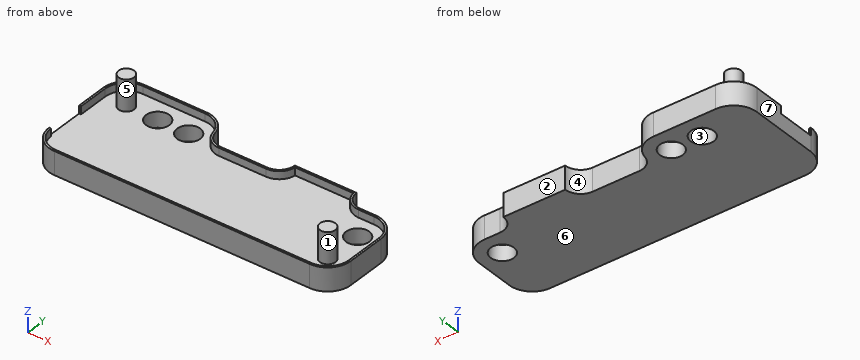
from build123d import *

# Parameters (mm, degrees)
SKETCH1_R           = 1
SKETCH1_R_2         = 1.5
BOSS_EXTRUDE1_DEPTH = 2
BOSS_EXTRUDE2_DEPTH = 3
SKETCH1_4_R         = 1
BOSS_EXTRUDE3_DEPTH = 6
SKETCH2_W           = 4
SKETCH2_H           = 5
CUT_EXTRUDE1_DEPTH  = 3


with BuildPart() as part:
    # Sketch1 → Boss-Extrude1 (new body)
    with BuildSketch(Plane.XY):
        with BuildLine():
            ThreePointArc((3, 0.25), (1.055456352, 1.055456352), (0.25, 3))
            Line((0.25, 3), (0.25, 12))
            ThreePointArc((0.25, 12), (1.055456352, 13.944543648), (3, 14.75))
            Line((3, 14.75), (11.060612309, 14.75))
            ThreePointArc((11.060612309, 14.75), (12.799865022, 14.13014084), (13.755051026, 12.55))
            ThreePointArc((13.755051026, 12.55), (14.536566847, 11.257157494), (15.959591794, 10.75))
            Line((15.959591794, 10.75), (22, 10.75))
            ThreePointArc((22, 10.75), (23.5, 11.322949017), (24.236067977, 12.75))
            Line((24.236067977, 12.75), (31.763932023, 12.75))
            ThreePointArc((31.763932023, 12.75), (32.5, 11.322949017), (34, 10.75))
            Line((34, 10.75), (36, 10.75))
            ThreePointArc((36, 10.75), (37.944543648, 9.944543648), (38.75, 8))
            Line((38.75, 8), (38.75, 3))
            ThreePointArc((38.75, 3), (37.944543648, 1.055456352), (36, 0.25))
            Line((36, 0.25), (3, 0.25))
        make_face()
        with Locations((36, 3)):
            Circle(SKETCH1_R, mode=Mode.SUBTRACT)
        with Locations((36, 8)):
            Circle(SKETCH1_R_2, mode=Mode.SUBTRACT)
        with Locations((3, 12)):
            Circle(SKETCH1_R, mode=Mode.SUBTRACT)
        with Locations((7.060612309, 12)):
            Circle(SKETCH1_R_2, mode=Mode.SUBTRACT)
        with Locations((11.060612309, 12)):
            Circle(SKETCH1_R_2, mode=Mode.SUBTRACT)
    extrude(amount=BOSS_EXTRUDE1_DEPTH)

    # Sketch1_3 → Boss-Extrude2 (add)
    with BuildSketch(Plane.XY):
        with BuildLine():
            Line((3, 0), (36, 0))
            ThreePointArc((36, 0), (38.121320344, 0.878679656), (39, 3))
            Line((39, 3), (39, 8))
            ThreePointArc((39, 8), (38.121320344, 10.121320344), (36, 11))
            Line((36, 11), (34, 11))
            ThreePointArc((34, 11), (32.585786438, 11.585786438), (32, 13))
            Line((32, 13), (24, 13))
            ThreePointArc((24, 13), (23.414213562, 11.585786438), (22, 11))
            Line((22, 11), (15.959591794, 11))
            ThreePointArc((15.959591794, 11), (14.69468073, 11.450806662), (14, 12.6))
            ThreePointArc((14, 12.6), (12.957978905, 14.323790008), (11.060612309, 15))
            Line((11.060612309, 15), (3, 15))
            ThreePointArc((3, 15), (0.878679656, 14.121320344), (0, 12))
            Line((0, 12), (0, 3))
            ThreePointArc((0, 3), (0.878679656, 0.878679656), (3, 0))
        make_face()
        with BuildLine():
            Line((3, 0.25), (36, 0.25))
            ThreePointArc((36, 0.25), (37.944543648, 1.055456352), (38.75, 3))
            Line((38.75, 3), (38.75, 8))
            ThreePointArc((38.75, 8), (37.944543648, 9.944543648), (36, 10.75))
            Line((36, 10.75), (34, 10.75))
            ThreePointArc((34, 10.75), (32.5, 11.322949017), (31.763932023, 12.75))
            Line((31.763932023, 12.75), (24.236067977, 12.75))
            ThreePointArc((24.236067977, 12.75), (23.5, 11.322949017), (22, 10.75))
            Line((22, 10.75), (15.959591794, 10.75))
            ThreePointArc((15.959591794, 10.75), (14.536566847, 11.257157494), (13.755051026, 12.55))
            ThreePointArc((13.755051026, 12.55), (12.799865022, 14.13014084), (11.060612309, 14.75))
            Line((11.060612309, 14.75), (3, 14.75))
            ThreePointArc((3, 14.75), (1.055456352, 13.944543648), (0.25, 12))
            Line((0.25, 12), (0.25, 3))
            ThreePointArc((0.25, 3), (1.055456352, 1.055456352), (3, 0.25))
        make_face(mode=Mode.SUBTRACT)
    extrude(amount=BOSS_EXTRUDE2_DEPTH)

    # Sketch1_4 → Boss-Extrude3 (add)
    with BuildSketch(Plane.XY):
        with Locations((3, 12)):
            Circle(SKETCH1_4_R)
        with Locations((36, 3)):
            Circle(SKETCH1_4_R)
    extrude(amount=BOSS_EXTRUDE3_DEPTH)

    # Sketch2 → Cut-Extrude1 (cut, symmetric)
    with BuildSketch(Plane.ZY):
        with Locations((4, 5.5)):
            Rectangle(SKETCH2_W, SKETCH2_H)
    extrude(amount=CUT_EXTRUDE1_DEPTH, both=True, mode=Mode.SUBTRACT)


solid = part.part
Input: part model. Units: mm. Frame: model coordinates. Face numbers are marked on the shaded views. A direction names the side the tool comes from. Round coordinates to 2 decimals unless told otherwise and drop trailing zeros. Order: outer loops, then holes, each group sorted by start corner. A loop starts at its lowest first (then second) coordinate and runs counter-clockwise, first axis right, second up.
1. Material intervals for line 1 (Y direction, x = 36, z = 2.5); line 2 (Y direction, x = 2.5, z = 2.5); line 3 (Y direction, x = 34.5, z = 2.45), sorted ascending.
The answers:
line 1: y = 0 to 0.25, 2 to 4, 10.75 to 11
line 2: y = 0.04 to 0.3, 11.13 to 12.87, 14.7 to 14.96
line 3: y = 0 to 0.25, 10.75 to 11
2. Mould query, pull axis X, two halves, no side actions, for the marked faces 5, 6 and 7. Classes: released by +X, released by -X, zero draft, split by the parting line, or undercut.
The answers:
face 5: undercut
face 6: zero draft
face 7: released by -X
3. Cut plane A-A, the plane z = 1.25. Output: boundary loops of the cut face in (x, y).
The answers:
outline: (0, 3) arc R3 ccw to (3, 0) - (36, 0) arc R3 ccw to (39, 3) - (39, 8) arc R3 ccw to (36, 11) - (34, 11) arc R2 cw to (32, 13) - (24, 13) arc R2 cw to (22, 11) - (15.96, 11) arc R2 cw to (14, 12.6) arc R3 ccw to (11.06, 15) - (3, 15) arc R3 ccw to (0, 12) - close; hole circle Ø3 at (7.06, 12); hole circle Ø3 at (11.06, 12); hole circle Ø3 at (36, 8)
4. Cut plane B-B, the plane x = 26.5. Output: boundary loops of the cut face in (y, z).
The answers:
outline: (0, 0) - (13, 0) - (13, 3) - (12.75, 3) - (12.75, 2) - (0.25, 2) - (0.25, 3) - (0, 3) - close
5. Pin query (flat end, axial travel): P1, Ø0.9, axis at x = 18.5, z = 2, coming from the +Y side; P2, Ø4, axis at x = 11.06, y = 12, coming from the +Z side; P3, Ø1, axis at x = 21.5, z = 5, coming from the -Y side; P4, Ø7.5, axis at x = 12, y = 9, coming from the +Z side. Return the tip coordinate at first contact, or that it passes through.
The answers:
P1: stops at y = 11
P2: stops at z = 2
P3: passes through
P4: stops at z = 3
6. Cut plane D-D, the plane z = 3.4. Output: boundary loops of the cut face in (x, y).
The answers:
outline: circle Ø2 at (3, 12); circle Ø2 at (36, 3)
7. Set-up query: the marked faces 1, 2, 3 and 4. Return all of +Z, -Z, +X, -X, +Y, -Y with unobstructed straight access to the full face (end or side cutting, diameter ignored); none if empty.
The answers:
face 1: +Z
face 2: +Z, -Z, +X, +Y
face 3: +Z, -Z
face 4: +Z, -Z, +Y
8. Cut plane C-C, the plane y = 9. Output: boundary loops of the cut face in (x, z), then the cut area to 3 significant figures.
The answers:
outline: (0, 0) - (34.88, 0) - (34.88, 2) - (0.25, 2) - (0.25, 3) - (0, 3) - close; (37.12, 0) - (38.83, 0) - (38.83, 3) - (38.56, 3) - (38.56, 2) - (37.12, 2) - close
area: 73.7 mm2
